from build123d import *

# Parameters (mm, degrees)
SKETCH_1_W           = 80
SKETCH_1_H           = 70
EXTRUDE_1_DEPTH      = 200
CUT_EXTRUDE_1_DEPTH  = 65
SKETCH_3_R           = 11
CUT_EXTRUDE_2_DEPTH  = 10
SKETCH_4_R           = 2
SKETCH_4_W           = 27
SKETCH_4_H           = 36
CUT_EXTRUDE_3_DEPTH  = 10
SKETCH_7_R           = 1.5
CUT_EXTRUDE_6_DEPTH  = 10
SKETCH_8_W           = 160
SKETCH_8_H           = 55
CUT_EXTRUDE_7_DEPTH  = 81
SKETCH_10_R          = 7
CUT_EXTRUDE_9_DEPTH  = 10
SKETCH_11_R          = 3
CUT_EXTRUDE_10_DEPTH = 10
SKETCH_12_R          = 2.555087711
CUT_EXTRUDE_11_DEPTH = 10
SKETCH_13_R          = 2
CUT_EXTRUDE_12_DEPTH = 20


with BuildPart() as part:
    # 草图1 → 凸台-拉伸1 (new body)
    with BuildSketch(Plane.XY):
        Rectangle(SKETCH_1_W, SKETCH_1_H)
    extrude(amount=-EXTRUDE_1_DEPTH)

    # 草图2 → 切除-拉伸1 (cut)
    with BuildSketch(Plane(origin=(0, 35, 0), x_dir=(1, 0, 0), z_dir=(0, 1, 0))):
        with BuildLine():
            ThreePointArc((-35, 192), (-34.121320344, 194.121320344), (-32, 195))
            Line((-32, 195), (32, 195))
            ThreePointArc((32, 195), (34.121320344, 194.121320344), (35, 192))
            Line((35, 192), (35, 8))
            ThreePointArc((35, 8), (34.121320344, 5.878679656), (32, 5))
            Line((32, 5), (-32, 5))
            ThreePointArc((-32, 5), (-34.121320344, 5.878679656), (-35, 8))
            Line((-35, 8), (-35, 192))
        make_face()
    extrude(amount=-CUT_EXTRUDE_1_DEPTH, mode=Mode.SUBTRACT)

    # 草图3 → 切除-拉伸2 (cut)
    with BuildSketch(Plane.XY):
        with Locations((0, 7)):
            Circle(SKETCH_3_R)
    extrude(amount=-CUT_EXTRUDE_2_DEPTH, mode=Mode.SUBTRACT)

    # 草图4 → 切除-拉伸3 (cut)
    with BuildSketch(Plane.ZY.offset(40)):
        with Locations((-121.5, 2)):
            Circle(SKETCH_4_R)
        with Locations((-121.5, 26)):
            Circle(SKETCH_4_R)
        with Locations((-158.5, 26)):
            Circle(SKETCH_4_R)
        with Locations((-158.5, 2)):
            Circle(SKETCH_4_R)
        with Locations((-140, 14)):
            Rectangle(SKETCH_4_W, SKETCH_4_H)
    extrude(amount=-CUT_EXTRUDE_3_DEPTH, mode=Mode.SUBTRACT)

    # 草图7 → 切除-拉伸6 (cut)
    with BuildSketch(Plane(origin=(0, 35, 0), x_dir=(1, 0, 0), z_dir=(0, 1, 0))):
        with Locations((-37, 150)):
            Circle(SKETCH_7_R)
        with Locations((-37, 50)):
            Circle(SKETCH_7_R)
        with Locations((37, 50)):
            Circle(SKETCH_7_R)
        with Locations((37, 150)):
            Circle(SKETCH_7_R)
        with Locations((0, 197)):
            Circle(SKETCH_7_R)
        with Locations((0, 3)):
            Circle(SKETCH_7_R)
    extrude(amount=-CUT_EXTRUDE_6_DEPTH, mode=Mode.SUBTRACT)

    # 草图8 → 切除-拉伸7 (cut, through all)
    with BuildSketch(Plane(origin=(40, 0, 0), x_dir=(0, 0, -1), z_dir=(1, 0, 0))):
        with Locations((100, 7.5)):
            Rectangle(SKETCH_8_W, SKETCH_8_H)
    extrude(amount=-CUT_EXTRUDE_7_DEPTH, mode=Mode.SUBTRACT)

    # 草图10 → 切除-拉伸9 (cut)
    with BuildSketch(Plane(origin=(0, 0, -200), x_dir=(-1, 0, 0), z_dir=(0, 0, -1))):
        with Locations((0, 7)):
            Circle(SKETCH_10_R)
    extrude(amount=-CUT_EXTRUDE_9_DEPTH, mode=Mode.SUBTRACT)

    # 草图11 → 切除-拉伸10 (cut)
    with BuildSketch(Plane(origin=(0, 0, -200), x_dir=(-1, 0, 0), z_dir=(0, 0, -1))):
        with Locations((-21.5, 7)):
            Circle(SKETCH_11_R)
        with Locations((26.5, 7)):
            Circle(SKETCH_11_R)
    extrude(amount=-CUT_EXTRUDE_10_DEPTH, mode=Mode.SUBTRACT)

    # 草图12 → 切除-拉伸11 (cut)
    with BuildSketch(Plane(origin=(0, 0, -200), x_dir=(-1, 0, 0), z_dir=(0, 0, -1))):
        with Locations((-25.052626778, -16)):
            Circle(SKETCH_12_R)
        with Locations((-25.052626778, 30)):
            Circle(SKETCH_12_R)
        with Locations((27, 30)):
            Circle(SKETCH_12_R)
        with Locations((27, -16)):
            Circle(SKETCH_12_R)
    extrude(amount=-CUT_EXTRUDE_11_DEPTH, mode=Mode.SUBTRACT)

    # 草图13 → 切除-拉伸12 (cut)
    with BuildSketch(Plane.XY):
        with Locations((25, -15)):
            Circle(SKETCH_13_R)
        with Locations((25, 29)):
            Circle(SKETCH_13_R)
        with Locations((-25, 29)):
            Circle(SKETCH_13_R)
        with Locations((-25, -15)):
            Circle(SKETCH_13_R)
    extrude(amount=-CUT_EXTRUDE_12_DEPTH, mode=Mode.SUBTRACT)


solid = part.part
Work out the finished part from the listing and answer in its coordinate system (mm). A direction names the side the tool comes from. Round coordinates to 2 decimals unless told otherwise and drop trailing zeros. Write each loop counter-clockwise with the first axis right and the second up, starting at its lowest first coordinate (ties: lowest second). Pieces come first, ordered by that corner, then holes. Notation, with made-up numbers: (2.25, -27) - (54.25, -27) arc R17 ccw to (54.25, -23) - close; hole circle Ø1 at (-23.75, 31). An arc over 180 degrees is marked (long way). Answer in a Markdown table with one row per item. Add a question column.
1. A cutting plane is placed at A-A, the plane y = -10. Determine the outline of the cut face in (x, z), and give its area (3 significant figures).
2. Given pin 1 (4 mm diameter, centred on x = -37, y = -4.5, fed in from +Z); pin 2 (1.5 mm diameter, centred on x = 23.5, z = -161, fed in from +Y); pin 3 (2.5 mm diameter, centred on x = 0, z = -197, fed in from +Y); pin 4 (4 mm diameter, centred on x = -37.5, z = -109, fed in from +Y), each flat-ended and moving along its own axis, determine where each tip first touches the part or whether it passes through.
3. The mould has two halves that part along Y. Classify faces 5 (the cylindrical face through (1.517, 0.166, -197.535)), 6 (the cylindrical face through (-25, 27, -2)), 7 (the flat face through (38, 7, -20)), 8 (the flat face through (3, 35, -196)): +Y half, -Y half, draft (parallel to the pull), parting line (faces both ways), or undercut.
4. A cutting plane is placed at D-D, the plane y = -2. Determine the outline of the cut face in (x, z), and give its area (3 significant figures).
5. A cutting plane is placed at B-B, the plane x = -4. Determine the outline of the cut face in (y, z).
6. A cutting plane is placed at C-C, the plane z = -81. Determine the outline of the cut face in (x, y), and give its area (3 significant figures).
7. Find the intervals of material crossed by line 1 along Y through (x, z) = (-25, -3.8); line 2 along Z through (x, y) = (0, 33); line 3 along X through (y, z) = (29.25, -3), in increasing order. Write a range as from..to.
8. For faces 1 (the cylindrical face through (25, 27, -2)), 2 (the flat face through (0, -30, -101)), 3 (the cylindrical face through (27.605, -15.888, -197.535)), 4 (the flat face through (-37, 7, -20)), determine the directions among +Z, -Z, +X, -X, +Y, -Y from which every point of the face is accessible in a straight line to the end or side of a thin tool.
Worked out:
| question | item | result |
|---|---|---|
| 1 | outline | (-40, -200) - (40, -200) - (40, -180) - (35, -180) - (35, -192) arc R3 cw to (32, -195) - (-32, -195) arc R3 cw to (-35, -192) - (-35, -180) - (-40, -180) - close; (-40, -20) - (-35, -20) - (-35, -8) arc R3 cw to (-32, -5) - (32, -5) arc R3 cw to (35, -8) - (35, -20) - (40, -20) - (40, 0) - (-40, 0) - close |
| 1 | area | 1,110 mm^2 |
| 2 | pin 1 | z = 0 |
| 2 | pin 2 | y = -30 |
| 2 | pin 3 | y = 25 |
| 2 | pin 4 | y = -20 |
| 3 | face 5 | undercut |
| 3 | face 6 | undercut |
| 3 | face 7 | draft |
| 3 | face 8 | +Y half |
| 4 | outline | (-40, -200) - (40, -200) - (40, -180) - (35, -180) - (35, -192) arc R3 cw to (32, -195) - (-32, -195) arc R3 cw to (-35, -192) - (-35, -180) - (-40, -180) - close; (-40, -20) - (-35, -20) - (-35, -8) arc R3 cw to (-32, -5) - (-6.32, -5) - (-6.32, 0) - (-40, 0) - close; (6.32, -5) - (32, -5) arc R3 cw to (35, -8) - (35, -20) - (40, -20) - (40, 0) - (6.32, 0) - close |
| 4 | area | 1,040 mm^2 |
| 5 | outline | (-35, -200) - (1.26, -200) - (1.26, -195) - (-30, -195) - (-30, -5) - (-3.25, -5) - (-3.25, 0) - (-35, 0) - close; (12.74, -200) - (35, -200) - (35, -195) - (12.74, -195) - close; (17.25, -5) - (35, -5) - (35, 0) - (17.25, 0) - close |
| 6 | outline | (-40, -35) - (40, -35) - (40, -20) - (35, -20) - (35, -30) - (-35, -30) - (-35, -20) - (-40, -20) - close |
| 6 | area | 500 mm^2 |
| 7 | line 1 | -35..-17, -13..27, 31..35 |
| 7 | line 2 | -200..-198.5, -195.5..-195, -5..-4.5, -1.5..0 |
| 7 | line 3 | -40..-26.98, -23.02..-1.5, 1.5..23.02, 26.98..40 |
| 8 | face 1 | +Z |
| 8 | face 2 | +Y |
| 8 | face 3 | -Z |
| 8 | face 4 | +X, -X, +Y |
